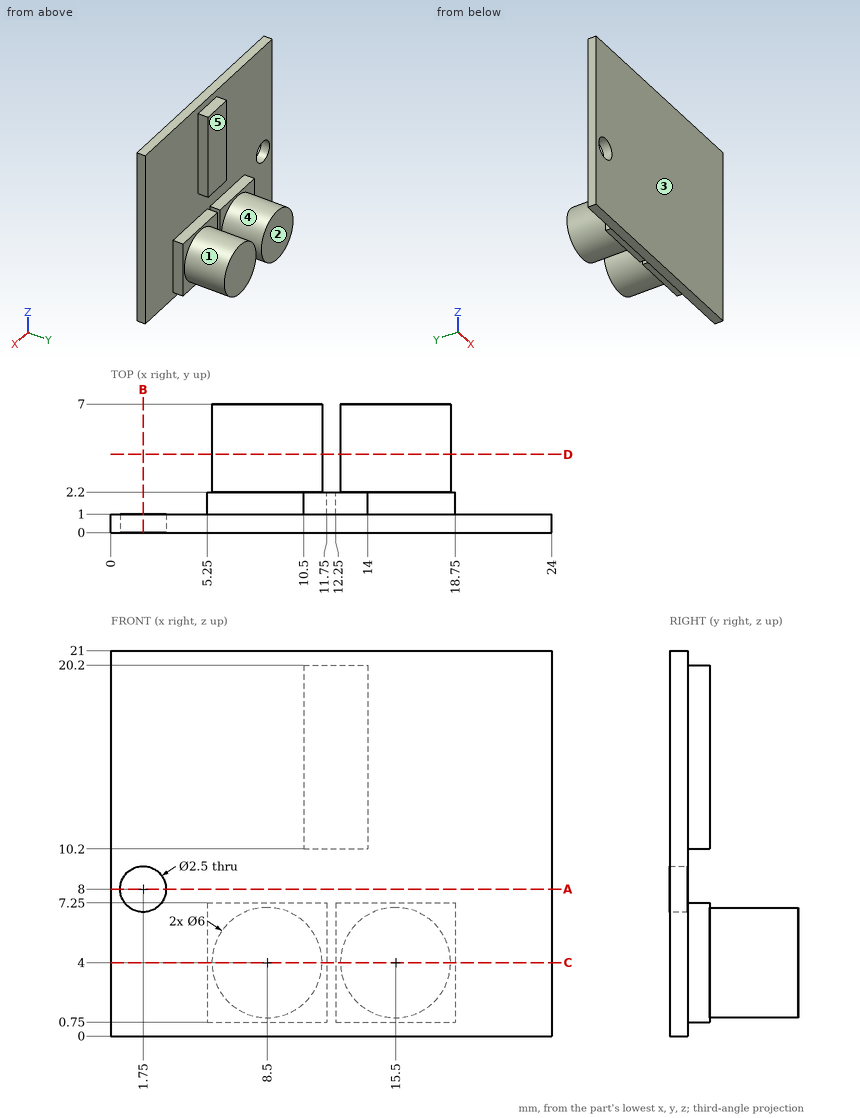
Geometry check sheet. Reference: drawing and pictorial views, mm from the part's lowest x, y, z. A direction names the side the tool comes from. Give positions to 0.01 mm unless a question says otherwise; leave off trailing zeros. Loops run counter-clockwise (first coordinate to the right, second up) from the corner with the lowest first, then second, coordinate; pieces in that order, holes last.
1. Go/stop test with flat-tipped pins: pin 1 Ø0.6 at (y, z) = (1.5, 14) entering from +X; pin 2 Ø8 at (x, z) = (10, 13) entering from +Y; pin 3 Ø1.5 at (x, y) = (15.5, 2) entering from +Z. Record where each tip stops, or that it passes through.
2. Thickness scan on line 1 (X direction, y = 0.3, z = 8); line 2 (Y direction, x = 7.5, z = 10); line 3 (X direction, y = 2, z = 17.25). Record the ranges inside material, lowest first.
3. Mould release check, pull along X, two halves, no side actions. Record for the marked faces 1 and 2: released by +X, released by -X, zero draft, split by the parting line, or undercut.
4. Section check D-D, the plane y = 4.25. Enter the section's corners in (x, z), then the cut area to 3 significant figures.
5. Section check A-A, the plane z = 8. Enter the section's corners in (x, y), then the cut area to 3 significant figures.
6. Section check C-C, the plane z = 4. Enter the section's corners in (x, y), then the cut area to 3 significant figures.
7. Set-up check for the marked faces 3, 4 and 5: record each of +Z, -Z, +X, -X, +Y, -Y from which the full face is reachable in a straight line by a thin tool's end or side.
8. Section check B-B, the plane x = 1.75. Enter the section's corners in (y, z), then the cut area to 3 significant figures.
Geometry says:
1. pin 1: stops at x = 14
1. pin 2: stops at y = 2.2
1. pin 3: stops at z = 7.25
2. line 1: x = 0 to 0.5, 3 to 24
2. line 2: y = 0 to 1
2. line 3: x = 10.5 to 14
3. face 1: undercut
3. face 2: zero draft
4. outline: circle Ø6 at (8.5, 4); circle Ø6 at (15.5, 4)
4. area: 56.5 mm2
5. outline: (0, 0) - (0.5, 0) - (0.5, 1) - (0, 1) - close; (3, 0) - (24, 0) - (24, 1) - (3, 1) - close
5. area: 21.5 mm2
6. outline: (0, 0) - (24, 0) - (24, 1) - (18.75, 1) - (18.75, 2.2) - (18.5, 2.2) - (18.5, 7) - (12.5, 7) - (12.5, 2.2) - (12.25, 2.2) - (12.25, 1) - (11.75, 1) - (11.75, 2.2) - (11.5, 2.2) - (11.5, 7) - (5.5, 7) - (5.5, 2.2) - (5.25, 2.2) - (5.25, 1) - (0, 1) - close
6. area: 97.2 mm2
7. face 3: +Z, -Z, +X, -X, -Y
7. face 4: +Y
7. face 5: +Z, +X, -X, +Y
8. outline: (0, 0) - (1, 0) - (1, 6.75) - (0, 6.75) - close; (0, 9.25) - (1, 9.25) - (1, 21) - (0, 21) - close
8. area: 18.5 mm2
